Could you check a few things on this model? Use its own coordinates, in mm. Face numbers are marked on the shaded views. A direction names the side the tool comes from. Give positions to 0.01 mm unless a question says otherwise; leave off trailing zeros. Order: outer loops, then holes, each group sorted by start corner. A loop starts at its lowest first (then second) coordinate and runs counter-clockwise, first axis right, second up. Notation, with made-up numbers: M -8,74.5 L 23,74.5 A25 ccw 23,109.5 Z; hole C 51.5,61.25 d2. An arc over 180 degrees is marked long. Answer in a Markdown table with one row per item. Add a question column.
```python
from build123d import *

# Parameters (mm, degrees)
SKETCH1_W           = 40
SKETCH1_H           = 4
SKETCH1_W_2         = 2
BOSS_EXTRUDE1_DEPTH = 3.7


with BuildPart() as part:
    # Sketch1 → Boss-Extrude1 (new body)
    with BuildSketch(Plane(origin=(0, 0, 0), x_dir=(1, 0, 0), z_dir=(0, 1, 0))):
        Polygon((-15.330595421, 3.400821374), (-17.330595421, 3.400821374), (-17.330595421, -0.599178626), (-15.330595421, -0.599178626), (24.669404579, -0.599178626), (24.669404579, 3.400821374), align=None)
        with Locations((4.669404579, -2.599178626)):
            Rectangle(SKETCH1_W, SKETCH1_H)
        with Locations((25.669404579, 1.400821374)):
            Rectangle(SKETCH1_W_2, SKETCH1_H)
        with Locations((4.669404579, 5.400821374)):
            Rectangle(SKETCH1_W, SKETCH1_H)
    extrude(amount=BOSS_EXTRUDE1_DEPTH)


solid = part.part
```
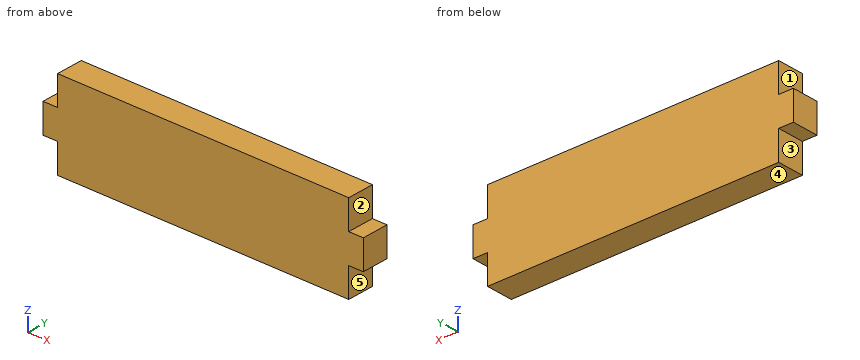
1. Suppose I cut it at B-B on z = 1.25. List the corners of the cut face in (x, y) for me.
2. Suppose I cut it at A-A on y = 2.9. List the corners of the cut face in (x, z) for me.
3. If I drill on line 1 along X through (y, z) = (0.3, -4), over which ranges is the centre line in solid material (lowest first)? Write a range as [from, to].
4. Will these pins go through, and if not, where does the flat tip stop? P1, Ø1.8, axis at y = 1, z = -5.5, coming from the +X side; P2, Ø1.1, axis at y = 1.5, z = 3.5, coming from the -X side; P3, Ø1.6, axis at x = -17, y = 2.5, coming from the +Z side.
5. For the marked faces 1, 2, 3, 4 and 5, which set-ups out of +Z, -Z, +X, -X, +Y, -Y let a thin tool reach every point of the face, with its end or its side?
Findings below:
| question | item | result |
|---|---|---|
| 1 | outline | M -15.33,0 L 24.67,0 L 24.67,3.7 L -15.33,3.7 Z |
| 2 | outline | M -17.33,-3.4 L -15.33,-3.4 L -15.33,-7.4 L 24.67,-7.4 L 24.67,-3.4 L 26.67,-3.4 L 26.67,0.6 L 24.67,0.6 L 24.67,4.6 L -15.33,4.6 L -15.33,0.6 L -17.33,0.6 Z |
| 3 | line 1 | [-15.33, 24.67] |
| 4 | P1 | x = 24.67 |
| 4 | P2 | x = -15.33 |
| 4 | P3 | z = 0.6 |
| 5 | face 1 | +Z, -X, +Y, -Y |
| 5 | face 2 | +Z, +X, +Y, -Y |
| 5 | face 3 | -Z, -X, +Y, -Y |
| 5 | face 4 | -Z, +X, -X, +Y, -Y |
| 5 | face 5 | -Z, +X, +Y, -Y |
